Here's how the part is built. I have some questions about the finished solid (model axes, mm). A direction names the side the tool comes from. Coordinates: 2 decimals unless noted, no trailing zeros. Loops run counter-clockwise (first coordinate to the right, second up) from the corner with the lowest first, then second, coordinate; pieces in that order, holes last.
```python
from build123d import *

# Parameters (mm, degrees)
BOSS_EXTRU_1_DEPTH      = 12
COQUE5_T                = -2
ENL_V_MAT_EXTRU_1_DEPTH = 2
BOSS_EXTRU_5_DEPTH      = 5


with BuildPart() as part:
    # Esquisse1 → Boss.-Extru.1 (new body)
    with BuildSketch(Plane.XY):
        with BuildLine():
            Line((5, 0), (47, 0))
            ThreePointArc((47, 0), (50.535533906, 1.464466094), (52, 5))
            Line((52, 5), (52, 32))
            ThreePointArc((52, 32), (50.535533906, 35.535533906), (47, 37))
            Line((47, 37), (5, 37))
            ThreePointArc((5, 37), (1.464466094, 35.535533906), (0, 32))
            Line((0, 32), (0, 5))
            ThreePointArc((0, 5), (1.464466094, 1.464466094), (5, 0))
        make_face()
    extrude(amount=BOSS_EXTRU_1_DEPTH)

    # Coque5
    coque5_openings = [part.faces().sort_by_distance(p)[0] for p in [
        (26, 18.5, 12),
    ]]
    offset(amount=COQUE5_T, openings=coque5_openings, kind=Kind.INTERSECTION)

    # Esquisse3 → Enlèv. mat.-Extru.1 (cut)
    with BuildSketch(Plane.XY.offset(12)):
        with BuildLine():
            ThreePointArc((51, 32), (49.828427125, 34.828427125), (47, 36))
            Line((47, 36), (5, 36))
            ThreePointArc((5, 36), (2.171572875, 34.828427125), (1, 32))
            Line((1, 32), (1, 5))
            ThreePointArc((1, 5), (2.171572875, 2.171572875), (5, 1))
            Line((5, 1), (47, 1))
            ThreePointArc((47, 1), (49.828427125, 2.171572875), (51, 5))
            Line((51, 5), (51, 32))
        make_face()
    extrude(amount=-ENL_V_MAT_EXTRU_1_DEPTH, mode=Mode.SUBTRACT)

    # Esquisse10 → Boss.-Extru.5 (add)
    # profile 1 of 2: a face of its own
    with BuildSketch(Plane(origin=(0, 0, 0), x_dir=(-1, 0, 0), z_dir=(0, 0, -1))):
        with BuildLine():
            Line((-40, 37), (-12, 37))
            Line((-12, 37), (-12, 43))
            ThreePointArc((-12, 43), (-12.585786438, 44.414213562), (-14, 45))
            Line((-14, 45), (-38, 45))
            ThreePointArc((-38, 45), (-39.414213562, 44.414213562), (-40, 43))
            Line((-40, 43), (-40, 37))
        make_face()
        with BuildLine():
            Line((-37.5, 39.5), (-37.5, 40.5))
            ThreePointArc((-37.5, 40.5), (-36.914213562, 41.914213562), (-35.5, 42.5))
            Line((-35.5, 42.5), (-16.5, 42.5))
            ThreePointArc((-16.5, 42.5), (-15.085786438, 41.914213562), (-14.5, 40.5))
            Line((-14.5, 40.5), (-14.5, 39.5))
            Line((-14.5, 39.5), (-37.5, 39.5))
        make_face(mode=Mode.SUBTRACT)
    # profile 2 of 2: a face of its own
    with BuildSketch(Plane(origin=(0, 0, 0), x_dir=(-1, 0, 0), z_dir=(0, 0, -1))):
        with BuildLine():
            Line((-40, 0), (-12, 0))
            Line((-12, 0), (-12, -6))
            ThreePointArc((-12, -6), (-12.585786438, -7.414213562), (-14, -8))
            Line((-14, -8), (-38, -8))
            ThreePointArc((-38, -8), (-39.414213562, -7.414213562), (-40, -6))
            Line((-40, -6), (-40, 0))
        make_face()
        with BuildLine():
            Line((-37.5, -2.5), (-37.5, -3.5))
            ThreePointArc((-37.5, -3.5), (-36.914213562, -4.914213562), (-35.5, -5.5))
            Line((-35.5, -5.5), (-16.5, -5.5))
            ThreePointArc((-16.5, -5.5), (-15.085786438, -4.914213562), (-14.5, -3.5))
            Line((-14.5, -3.5), (-14.5, -2.5))
            Line((-14.5, -2.5), (-37.5, -2.5))
        make_face(mode=Mode.SUBTRACT)
    extrude(amount=-BOSS_EXTRU_5_DEPTH)


solid = part.part
```
1. I need wall thicknesses on line 1 along Y through (x, z) = (29.5, 0.5); line 2 along Y through (x, z) = (16.5, 3.25); line 3 along Y through (x, z) = (21.5, 9.5). Which ranges of each line are inside material? Lowest first, please.
2. I want a section at C-C (z = 1). Give the number of separate pieces and of enclosed holes in the cut face, then the cut area to 3 significant figures.
3. For pin 1 (1.1 mm diameter, centred on y = -3, z = 1.5, fed in from -X); pin 2 (1 mm diameter, centred on x = 15.5, y = 21, fed in from +Z); pin 3 (5 mm diameter, centred on x = 19, z = 9.5, fed in from -Y), each with a flat end and sliding along its axis, tell me the tip position at first contact or that it passes through.
4. I want a section at B-B (y = 13). Please give me the cut outline in (x, z), then the cut area to 3 significant figures.
5. I want a section at A-A (x = 31). Please give me the cut outline in (y, z), then the cut area to 3 significant figures.
6. On a 3-axis mill with a long thin cutter (end or side, diameter ignored), from which of +Z, -Z, +X, -X, +Y, -Y can I reach the whole of each face in a straight line? I mean faces 4 (the flat face through (26, -6, 5)), 5 (the cylindrical face through (2.86, 2.9, 5.94)), 6 (the flat face through (26, 39.5, 2)), 7 (the flat face through (12, -3, 2)). Say none if no direction works.
7. We'd pull the mould along Y, two halves only. Please class faces 1 (the cylindrical face through (1, 2, 6)), 2 (the flat face through (2, 19, 6)), 3 (the flat face through (40, -3, 2)): +Y half, -Y half, draft (parallel to the pull), parting line (faces both ways), or undercut.
8. I want a section at D-D (x = 48). Please give me the cut outline in (y, z), then the cut area to 3 significant figures.
Response values:
1. line 1: y = -8 to -5.5, -2.5 to 39.5, 42.5 to 45
1. line 2: y = -8 to -5.5, -2.5 to 2, 35 to 39.5, 42.5 to 45
1. line 3: y = 0 to 2, 35 to 37
2. separate pieces: 1
2. enclosed holes: 2
2. area: 2,210 mm2
3. pin 1: stops at x = 12
3. pin 2: stops at z = 2
3. pin 3: stops at y = 0
4. outline: (0, 0) - (52, 0) - (52, 12) - (51, 12) - (51, 10) - (50, 10) - (50, 2) - (2, 2) - (2, 10) - (1, 10) - (1, 12) - (0, 12) - close
4. area: 140 mm2
5. outline: (-8, 0) - (-5.5, 0) - (-5.5, 5) - (-8, 5) - close; (-2.5, 0) - (39.5, 0) - (39.5, 5) - (37, 5) - (37, 12) - (36, 12) - (36, 10) - (35, 10) - (35, 2) - (2, 2) - (2, 10) - (1, 10) - (1, 12) - (0, 12) - (0, 5) - (-2.5, 5) - close; (42.5, 0) - (45, 0) - (45, 5) - (42.5, 5) - close
5. area: 160 mm2
6. face 4: +Z, +X, -X, -Y
6. face 5: +Z
6. face 6: +Z, -Z
6. face 7: +Z, -Z, -X, -Y
7. face 1: -Y half
7. face 2: undercut
7. face 3: draft
8. outline: (0.1, 0) - (36.9, 0) - (36.9, 12) - (35.87, 12) - (35.87, 10) - (34.83, 10) - (34.83, 2) - (2.17, 2) - (2.17, 10) - (1.13, 10) - (1.13, 12) - (0.1, 12) - close
8. area: 111 mm2
